Model file for the job. Use its own axes, mm. Coordinates: 2 decimals unless noted, no trailing zeros. Write each loop counter-clockwise with the first axis right and the second up, starting at its lowest first coordinate (ties: lowest second). Pieces come first, ordered by that corner, then holes. Notation, with made-up numbers: M 78,43 L 129,43 A17 ccw 129,48 Z; hole C 6,88 d11. An arc over 180 degrees is marked long. One line per question, with ' | ' between items. Start each with the question number.
(1) Cut at B-B (z = 341.5). Write the cut outline in (x, y).
(2) Two-plate mould, pull along Y, no slides. Class faces 1 (the face through (-172.434, 166.696, 234.643)), 2 (the face through (-181.996, 69.123, 280.965)), 3 (the face through (-184.996, 69.123, 280.965)): +Y half, -Y half, draft (parallel to the pull), parting line (faces both ways), or undercut.
(3) Cut at A-A (z = 263). Write the cut outline in (x, y), plus the area to 3 significant figures.
(4) Cut at D-D (y = 86). Write the cut outline in (x, z).
(5) Wall check: probe 1 along X at (y, z) = (126.5, 321); probe 2 along X at (y, z) = (73.5, 262). Give the ranges that are in metal, low to high.
(6) Cut at C-C (y = 119.5). Write the cut outline in (x, z), plus the area to 3 significant figures.
(7) Flat gauge pins, fed straight in: pin 1 Ø10 at (x, z) = (-186, 289) entering from -Y; pin 2 Ø5 at (x, y) = (-163.5, 195) entering from -Z; pin 3 Ø6 at (x, y) = (-181, 100.5) entering from +Z. Where does each tip first touch, or does it go through?
from build123d import *

# Parameters (mm, degrees)
BOSS_EXTRUDE1_DEPTH = 3
SKETCH1_R           = 2.5
BOSS_EXTRUDE2_DEPTH = 3
BOSS_EXTRUDE5_DEPTH = 3


with BuildPart() as part:
    # 3DSketch1 → Boss-Extrude1 (new, along a direction that is not the sketch's normal)
    with BuildSketch(Plane(origin=(-191.853103939, 23, 196.386082525), x_dir=(0.06876662353575062, 0.5251074950069344, 0.8482530696525858), z_dir=(0.9967300562972695, 0, -0.08080343355106794))):
        Polygon((0, 0), (137.697420516, 85.103590916), (190.208170017, 0), (47.360694134, -76.756953147), align=None)
    extrude(amount=BOSS_EXTRUDE1_DEPTH, dir=(1, 0, 0))

    # Sketch1 → Boss-Extrude2 (add)
    with BuildSketch(Plane(origin=(0, 23.146370891, 0.017253018), x_dir=(1, 0, 0), z_dir=(0, -0.9999997221987764, -0.000745387395963266))):
        Polygon((-175.773130318, 357.71359297), (-167.773130318, 357.71359297), (-180.853103939, 196.301655796), (-188.853103939, 196.301655796), align=None)
        with Locations(Location((-172.434519968, 349.71359297, 0), (0, 0, 270))):
            Circle(SKETCH1_R, mode=Mode.SUBTRACT)
        with Locations(Location((-184.217937823, 204.301655796, 0), (0, 0, 270))):
            Circle(SKETCH1_R, mode=Mode.SUBTRACT)
    extrude(amount=-BOSS_EXTRUDE2_DEPTH)

    # 3DSketch2 → Boss-Extrude5 (add, along a direction that is not the sketch's normal)
    with BuildSketch(Plane(origin=(-189.258816585, 115.113773206, 228.387249638), x_dir=(0.08065912513094323, 0.05973817293580263, 0.99494997674627), z_dir=(-0.9586958466573331, 0.27780635378188856, 0.06104017857437458))):
        Polygon((0, 0), (21.385713883, 107.795899991), (130, 0), align=None)
    extrude(amount=-BOSS_EXTRUDE5_DEPTH, dir=(-1, 0, 0))


solid = part.part
Filled in:
1) outline: M -180.09,22.89 L -177.09,22.89 L -177.09,121.91 L -172.9,136.36 L -175.9,136.36 L -180.09,121.91 Z; M -177.09,22.89 L -169.09,22.89 L -169.09,25.89 L -177.09,25.89 Z
2) face 1: +Y half | face 2: undercut | face 3: draft
3) outline: M -186.45,22.95 L -183.45,22.95 L -183.45,117.19 L -159.01,201.54 L -162.01,201.54 L -186.45,117.19 Z; M -183.45,22.95 L -175.45,22.95 L -175.45,25.95 L -183.45,25.95 Z | area: 560 mm²
4) outline: M -191.85,196.39 L -188.85,196.39 L -175.77,357.73 L -178.77,357.73 Z
5) probe 1: -180.06 to -177.06 | probe 2: -186.53 to -183.53
6) outline: M -187.95,228.92 L -184.95,228.92 L -180.34,301.44 L -175.77,357.73 L -178.77,357.73 L -183.34,301.44 Z | area: 386 mm²
7) pin 1: y = 22.93 | pin 2: z = 237.77 | pin 3: z = 357.73
